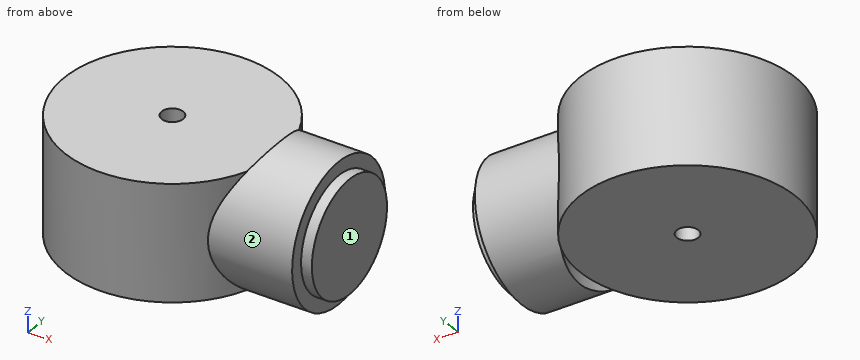
```python
from build123d import *

# Parameters (mm, degrees)
SKETCH1_R                = 50
BOSS_EXTRUDE1_DEPTH      = 54
BOSS_EXTRUDE2_REACH      = 148.782
BOSS_EXTRUDE2_END_RADIUS = 50
SKETCH3_R                = 32.5
SKETCH4_R                = 26.25
BOSS_EXTRUDE3_DEPTH      = 5
SKETCH5_R                = 5
CUT_EXTRUDE1_DEPTH       = 500


with BuildPart() as part:
    # Sketch1 → Boss-Extrude1 (new body)
    with BuildSketch(Plane.XY):
        Circle(SKETCH1_R)
    extrude(amount=BOSS_EXTRUDE1_DEPTH)

    # Boss-Extrude2: up to this cylinder (the profile starts outside it)
    boss_extrude2_end = Plane(origin=(0, 0, 27), z_dir=(0, 0, -1)) * Cylinder(BOSS_EXTRUDE2_END_RADIUS, 398.564, mode=Mode.PRIVATE)
    # Sketch3 → Boss-Extrude2 (add, up to the surface)
    with BuildSketch(Plane(origin=(77, 0, 0), x_dir=(0, 0, -1), z_dir=(1, 0, 0)), mode=Mode.PRIVATE) as boss_extrude2_sk1:
        with Locations((-27, 0)):
            Circle(SKETCH3_R)
    boss_extrude2_tool1 = extrude(boss_extrude2_sk1.sketch, amount=-BOSS_EXTRUDE2_REACH, mode=Mode.PRIVATE) - boss_extrude2_end
    add(boss_extrude2_tool1.solids().sort_by_distance((77, 0, 27))[0])

    # Sketch4 → Boss-Extrude3 (add)
    with BuildSketch(Plane(origin=(77, 0, 0), x_dir=(0, 0, -1), z_dir=(1, 0, 0))):
        with Locations((-27, 0)):
            Circle(SKETCH4_R)
    extrude(amount=BOSS_EXTRUDE3_DEPTH)

    # Sketch5 → Cut-Extrude1 (cut)
    with BuildSketch(Plane.XY.offset(54)):
        Circle(SKETCH5_R)
    extrude(amount=-CUT_EXTRUDE1_DEPTH, mode=Mode.SUBTRACT)


solid = part.part
```
Work out the finished part from the listing and answer in its coordinate system (mm). Face numbers are marked on the shaded views. A direction names the side the tool comes from. Round coordinates to 2 decimals unless told otherwise and drop trailing zeros. Write each loop counter-clockwise with the first axis right and the second up, starting at its lowest first coordinate (ties: lowest second). Pieces come first, ordered by that corner, then holes. Notation, with made-up numbers: (37.25, 5) -> (63.25, 5) arc R31 ccw to (63.25, 36) -> close; hole circle Ø8 at (69, -33). An arc over 180 degrees is marked (long way). Write each question's results on one line, items separated by ' | '.
1) Consider line 1 along Y through (x, z) = (0, 15); line 2 along Z through (x, y) = (-44, 5); line 3 along Y through (x, z) = (-2.5, 22). Determine where each line is inside the solid, lowest interval first. Write a range as [from, to].
Findings:
line 1: y = [-50, -5], [5, 50] | line 2: z = [0, 54] | line 3: y = [-49.94, -4.33], [4.33, 49.94]
2) The part is cut by section C-C (z = 23.5). Write down the section's boundary in (x, y).
Findings:
outline: (38.16, -32.31) -> (77, -32.31) -> (77, -26.02) -> (82, -26.02) -> (82, 26.02) -> (77, 26.02) -> (77, 32.31) -> (38.16, 32.31) arc R50 ccw (long way) to start; hole circle Ø10 at (0, 0)
3) The part is cut by section B-B (x = 0). Write down the section's boundary in (y, z).
Findings:
outline: (-50, 0) -> (-5, 0) -> (-5, 54) -> (-50, 54) -> close; (5, 0) -> (50, 0) -> (50, 54) -> (5, 54) -> close
4) The part is cut by section A-A (y = 0). Write down the section's boundary in (x, z), and give its area (3 significant figures).
Findings:
outline: (-50, 0) -> (-5, 0) -> (-5, 54) -> (-50, 54) -> close; (5, 0) -> (50, 0) -> (50, -5.5) -> (77, -5.5) -> (77, 0.75) -> (82, 0.75) -> (82, 53.25) -> (77, 53.25) -> (77, 59.5) -> (50, 59.5) -> (50, 54) -> (5, 54) -> close | area: 6,880 mm²
5) Which of the six approach directions +Z, -Z, +X, -X, +Y, -Y give full straight-line access (tool end or side, diameter ignored) to the marked faces 1 and 2?
Findings:
face 1: +Z, -Z, +X, +Y, -Y | face 2: +X
6) The part is cut by section D-D (x = 71.5). Write down the section's boundary in (y, z), and give its area (3 significant figures).
Findings:
outline: circle Ø65 at (0, 27) | area: 3,320 mm²
7) Flat-ended cylindrical pins translate along their axes: pin 1 (10 mm diameter, centred on y = -17, z = 40, fed in from -X); pin 2 (3 mm diameter, centred on y = 31.5, z = 38, fed in from +X); pin 3 (13 mm diameter, centred on x = 0, y = 0, fed in from +Z). Find the tip coordinate at first contact, or state that the pin passes through.
Findings:
pin 1: stops at x = -48.54 | pin 2: stops at x = 77 | pin 3: stops at z = 54
